Check sheet for the modelled part. Datum: model origin and axes. Units: mm. Face numbers are marked on the shaded views. Give positions to 0.01 mm unless a question says otherwise; leave off trailing zeros. Loops run counter-clockwise (first coordinate to the right, second up) from the corner with the lowest first, then second, coordinate; pieces in that order, holes last. Notation, with made-up numbers: (-31.5, 71.25) - (6.5, 71.25) arc R22 ccw to (6.5, 85.25) - close; hole circle Ø8 at (79.25, 35). An arc over 180 degrees is marked (long way). Answer in a Markdown table with one row per item. Add a question column.
(1) Go/stop test with flat-tipped pins: P1, Ø8, axis at x = 72, y = -10, coming from the +Z side; P2, Ø4, axis at x = 117, z = 19.5, coming from the +Y side. Record where each tip stops, or that it passes through.
(2) Thickness scan on L1, parallel to Y at x = 88.5, z = 15; L2, parallel to Z at x = 104, y = -3.2; L3, parallel to Z at x = 91, y = -13. Record the ranges inside material, lowest first.
(3) Sectioned sample at C-C on y = -9.5. Enter the section's corners in (x, z).
(4) Draft check along Z on the marked faces 1, 2 and 3. Enter one of: released by +Z, released by -Z, zero draft, split by the parting line, or undercut.
(5) Sectioned sample at A-A on z = 60. Enter the section's corners in (x, y), then the cut area to 3 significant figures.
(6) Sectioned sample at D-D on x = 163. Enter the section's corners in (y, z), then the cut area to 3 significant figures.
(7) Sectioned sample at B-B on x = 104. Enter the section's corners in (y, z).
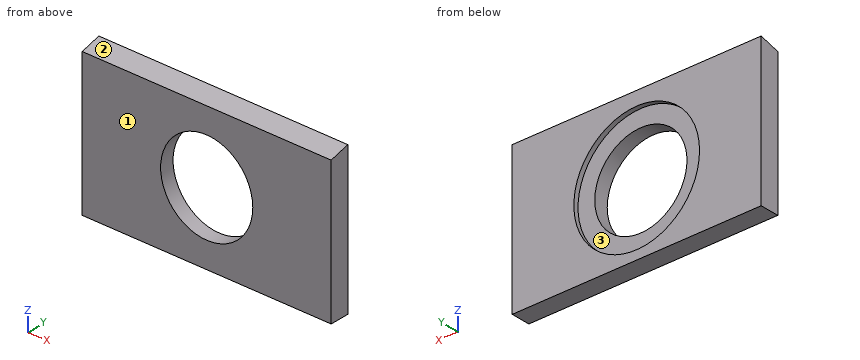
from build123d import *

# Parameters (mm, degrees)
F0_W     = 208
F0_H     = 124
F1_DEPTH = 16
F3_DEPTH = 240
F5_D     = 77
F6_R     = 52.5
F7_DEPTH = 4


with BuildPart() as f1:
    # F0 (on Front) → F1 (new body)
    with BuildSketch(Plane.XZ):
        with Locations((104, 62)):
            Rectangle(F0_W, F0_H)
    extrude(amount=F1_DEPTH)

    # F2 (on Right) → F3 (cut)
    with BuildSketch(Plane.YZ):
        Polygon((-16, 119.712813), (0, 124), (-16, 124), align=None)
    extrude(amount=F3_DEPTH, mode=Mode.SUBTRACT)

    # F5 (through all)
    with Locations(Plane(origin=(0, 0, 0), x_dir=(-1, 0, 0), z_dir=(0, 1, 0))):
        with Locations((-104, 60)):
            Hole(F5_D / 2)

    # F6 (on face) → F7 (cut)
    with BuildSketch(Plane(origin=(0, 0, 0), x_dir=(-1, 0, 0), z_dir=(0, 1, 0))):
        with Locations((-104, 60)):
            Circle(F6_R)
    extrude(amount=-F7_DEPTH, mode=Mode.SUBTRACT)


solid = f1.part
Reply:
| question | item | result |
|---|---|---|
| 1 | P1 | z = 122.39 |
| 1 | P2 | y = -4 |
| 2 | L1 | -16 to -4 |
| 2 | L2 | 0 to 7.5, 112.5 to 123.14 |
| 2 | L3 | 0 to 23.76, 96.24 to 120.52 |
| 3 | outline | (0, 0) - (208, 0) - (208, 121.45) - (0, 121.45) - close; hole circle Ø77 at (104, 60) |
| 4 | face 1 | zero draft |
| 4 | face 2 | released by +Z |
| 4 | face 3 | undercut |
| 5 | outline | (0, -16) - (65.5, -16) - (65.5, -4) - (51.5, -4) - (51.5, 0) - (0, 0) - close; (142.5, -16) - (208, -16) - (208, 0) - (156.5, 0) - (156.5, -4) - (142.5, -4) - close |
| 5 | area | 1,980 mm^2 |
| 6 | outline | (-16, 0) - (0, 0) - (0, 124) - (-16, 119.71) - close |
| 6 | area | 1,950 mm^2 |
| 7 | outline | (-16, 0) - (0, 0) - (0, 7.5) - (-4, 7.5) - (-4, 21.5) - (-16, 21.5) - close; (-16, 98.5) - (-4, 98.5) - (-4, 112.5) - (0, 112.5) - (0, 124) - (-16, 119.71) - close |
